Can you work these out from the model? Positions are in its coordinate system, mm. Face numbers are marked on the shaded views. A direction names the side the tool comes from. Round coordinates to 2 decimals unless told otherwise and drop trailing zeros. Loops run counter-clockwise (first coordinate to the right, second up) from the corner with the lowest first, then second, coordinate; pieces in that order, holes last.
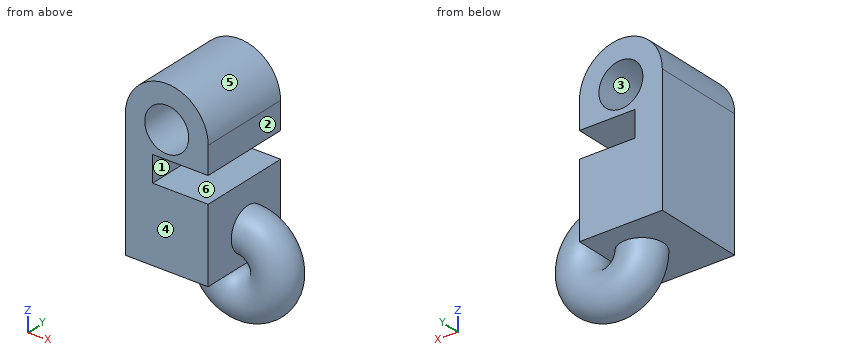
from build123d import *

# Parameters (mm, degrees)
F0_R     = 15.063186
F1_DEPTH = 63.5
F2_W     = 63.5
F2_H     = 17.738506
F3_DEPTH = 38.1
F4_R     = 14.591835


with BuildPart() as f1:
    # F0 (on Front) → F1 (new body)
    with BuildSketch(Plane.XZ):
        with BuildLine():
            Line((-28.397631, -43.692742), (28.397631, -43.692742))
            Line((28.397631, -43.692742), (28.397631, 43.692742))
            ThreePointArc((28.397631, 43.692742), (0, 72.090372), (-28.397631, 43.692742))
            Line((-28.397631, 43.692742), (-28.397631, -43.692742))
        make_face()
        with Locations((0, 43.692742)):
            Circle(F0_R, mode=Mode.SUBTRACT)
    extrude(amount=F1_DEPTH)

    # F2 (on face) → F3 (cut)
    with BuildSketch(Plane.YZ.offset(28.397631)):
        with Locations((-31.75, 16.151376)):
            Rectangle(F2_W, F2_H)
    extrude(amount=-F3_DEPTH, mode=Mode.SUBTRACT)

    # F4 (on face) → F5 (revolve)
    with BuildSketch(Plane.YZ.offset(28.397631)):
        with Locations((-28.650237, -23.23292)):
            Circle(F4_R)
    revolve(axis=Axis((28.397631, -31.75, -43.692742), (0, -1, 0)))


solid = f1.part
(1) If we section it at B-B, the plane z = 34.5: List the corners of the cut face in (x, y) for me, then the cut area to 3 significant figures.
Worked answers:
outline: (-28.4, -63.5) - (-11.93, -63.5) - (-11.93, 0) - (-28.4, 0) - close; (11.93, -63.5) - (28.4, -63.5) - (28.4, 0) - (11.93, 0) - close
area: 2,090 mm2
(2) If we mould it in two halves opening along Z, with no side actions, what happens to the marked faces 4, 5 and 6? For each: released by +Z, released by -Z, zero draft, split by the parting line, or undercut.
Worked answers:
face 4: zero draft
face 5: released by +Z
face 6: undercut
(3) If I drill on line 1 (Z direction, x = 0, y = -14); line 2 (Z direction, x = -1, y = -23); line 3 (X direction, y = -21.5, z = 8.5), over which ranges is the centre line in solid material (lowest first)?
Worked answers:
line 1: z = -43.69 to 7.28, 25.02 to 28.63, 58.76 to 72.09
line 2: z = -60.6 to 7.28, 25.02 to 28.66, 58.72 to 72.07
line 3: x = -28.4 to -9.7
(4) If we section it at C-C, the plane y = -49.5: List the corners of the cut face in (x, z) for me.
Worked answers:
outline: (-28.4, -43.69) - (28.4, -43.69) - (28.4, 7.28) - (-9.7, 7.28) - (-9.7, 25.02) - (28.4, 25.02) - (28.4, 43.69) arc R28.4 ccw to (-28.4, 43.69) - close; hole circle Ø30.13 at (0, 43.69)
(5) If we section it at A-A, the plane y = -24.5: List the corners of the cut face in (x, z) for me.
Worked answers:
outline: (-28.4, -43.69) - (-6.05, -43.69) arc R34.45 ccw (long way) to (28.4, -9.24) - (28.4, 7.28) - (-9.7, 7.28) - (-9.7, 25.02) - (28.4, 25.02) - (28.4, 43.69) arc R28.4 ccw to (-28.4, 43.69) - close; hole circle Ø30.13 at (0, 43.69); hole (21.93, -43.69) arc R6.47 ccw (long way) to (28.4, -37.22) - (28.4, -43.69) - close
(6) For the marked faces 1, 2 and 3, which set-ups out of +Z, -Z, +X, -X, +Y, -Y let a thin tool reach every point of the face, with its end or its side?
Worked answers:
face 1: +X, +Y, -Y
face 2: +Z, +X, +Y, -Y
face 3: +Y, -Y
(7) If we section it at D-D, the plane x = 11: State how many separate pieces and enclosed holes the cut face has, then the cut area to 3 significant figures.
Worked answers:
separate pieces: 3
enclosed holes: 0
area: 5,550 mm2
(8) Will these pins go through, and if not, where does the flat tip stop? P1, Ø11.5, axis at x = 13.5, y = -34, coming from the -Z side; P2, Ø3, axis at x = 51, y = -19, coming from the +Z side; P3, Ø19.5, axis at y = -42.5, z = 20.5, coming from the +X side; P4, Ø4, axis at x = 18, z = 28, coming from the +Y side.
Worked answers:
P1: stops at z = -77.09
P2: stops at z = -19.68
P3: stops at x = 28.4
P4: stops at y = 0
